Autodesk Inventor part; units mm, degrees
ref_plane "YZ Plane" through (0, 0, 0) normal (1, 0, 0) x (0, 1, 0)
ref_plane "XZ Plane" through (0, 0, 0) normal (0, 1, 0) x (-1, 0, 0)
ref_plane "XY Plane" through (0, 0, 0) normal (0, 0, 1) x (1, 0, 0)
sketch "Sketch1" plane through (0, 0, 0) normal (0, 0, 1) x (1, 0, 0)
  circle A0 centre (0, 12.7) radius 1.5875
  circle A1 centre (-0.0751, 0) radius 1.5875
  line L0 (-0.0751, 0) -> (-0.0751, 19.0499)
  line L1 (-0.0751, 1.5875) -> (-0.0751, 24.8386)
  line L2 (6.35, 15.5543) -> (6.35, 5.2605)
  line L3 (9.525, 2.0855) -> (15.8376, 2.0855)
  line L4 (-6.5001, 15.5229) -> (-6.5001, 5.2772)
  line L5 (-9.6751, 2.1022) -> (-15.8387, 2.1022)
  arc A2 (-19.0064, -1.2874) -> (19.0051, -1.3074) centre (0, 0) ccw
  arc A3 (3.81, 18.6651) -> (-3.9901, 18.6274) centre (0, 0) ccw
  arc A4 (-3.9901, 18.6274) -> (-6.5001, 15.5229) centre (-3.3251, 15.5229) ccw
  arc A5 (6.35, 15.5543) -> (3.81, 18.6651) centre (3.175, 15.5543) ccw
  arc A6 (6.35, 5.2605) -> (9.525, 2.0855) centre (9.525, 5.2605) ccw
  arc A7 (-9.6751, 2.1022) -> (-6.5001, 5.2772) centre (-9.6751, 5.2772) ccw
  arc A8 (-15.8387, 2.1022) -> (-19.0064, -1.2874) centre (-15.8387, -1.0728) ccw
  arc A9 (19.0051, -1.3074) -> (15.8376, 2.0855) centre (15.8376, -1.0895) ccw
  point P0 (6.35, 17.9605)
  point P1 (6.35, 2.0855)
  point P2 (18.9355, 2.0855)
  point P3 (-6.5001, 2.1022)
  point P4 (-18.9337, 2.1022)
  point P5 (-6.5001, 17.9067)
  dimension "d6" = 3.175
  dimension "d3" = 3.175
  dimension "d11" = 15.875
  dimension "d12" = 3.175
extrude "Extrusion1" add sketch "Sketch1" along normal blind 12.7
properties part number "Crank Cutting Jig"
Build history of the part. All positions in model axes, mm. A direction names the side the tool comes from. Coordinates: 2 decimals unless noted, no trailing zeros. Write each loop counter-clockwise with the first axis right and the second up, starting at its lowest first coordinate (ties: lowest second). Pieces come first, ordered by that corner, then holes.
(1) 3-axis set-ups, long thin cutter, end or side, ignore diameter. For faces 4 (the cylindrical face through (0.391, -19.046, 6.261)), 5 (the flat face through (-6.5, 10, 6)), 6 (the flat face through (13, 2.086, 6)): which of +Z, -Z, +X, -X, +Y, -Y reach the whole face in a straight line?
(2) Cut at B-B on z = 7. State how many separate pieces and enclosed holes the cut face has, and give its area (3 significant figures).
(3) Cut at C-C on x = 0. List the corners of the cut face in (y, z), and give its area (3 significant figures).
(4) Pin check, flat tips, straight feed: pin 1 Ø1.5 at (y, z) = (-5.5, 9.5) entering from -X; pin 2 Ø5 at (x, y) = (0, 12.7) entering from -Z; pin 3 Ø4 at (x, y) = (10, 8.5) entering from +Z; pin 4 Ø5 at (y, z) = (9.5, 4.5) entering from -X. Stop position of each tip, or through.
(5) Mould opens along X. For faces 1 (the cylindrical face through (7.305, 2.991, 6.261)), 2 (the flat face through (-13, 2.102, 6)), 3 (the cylindrical face through (1.44, -0.48, 6.26)) say: pulls with the +X half, pulls with the -X half, needs draft (parallel to the pull), parting line crosses it, or undercut.
(6) Cut at D-D on y = 0. List the corners of the cut face in (x, z).
(7) Cut at A-A on y = 12.7. List the corners of the cut face in (x, z), and give its area (3 significant figures).
(8) Drill centre lines: line 1 (Y direction, x = 0, z = 7.5); line 2 (X direction, y = 12.7, z = 2.75); line 3 (Y direction, x = 1, z = 8). Where is each one in solid material? Low to high.
Working result:
1. face 4: +Z, -Z, -Y
1. face 5: +Z, -Z, -X, +Y
1. face 6: +Z, -Z, +X, +Y
2. separate pieces: 1
2. enclosed holes: 2
2. area: 845 mm2
3. outline: (-19.05, 0) - (-1.59, 0) - (-1.59, 12.7) - (-19.05, 12.7) - close; (1.59, 0) - (11.11, 0) - (11.11, 12.7) - (1.59, 12.7) - close; (14.29, 0) - (19.05, 0) - (19.05, 12.7) - (14.29, 12.7) - close
3. area: 403 mm2
4. pin 1: stops at x = -18.45
4. pin 2: stops at z = 0
4. pin 3: passes through
4. pin 4: stops at x = -6.5
5. face 1: pulls with the +X half
5. face 2: needs draft
5. face 3: undercut
6. outline: (-18.83, 0) - (-1.66, 0) - (-1.66, 12.7) - (-18.83, 12.7) - close; (1.51, 0) - (18.82, 0) - (18.82, 12.7) - (1.51, 12.7) - close
7. outline: (-6.5, 0) - (-1.59, 0) - (-1.59, 12.7) - (-6.5, 12.7) - close; (1.59, 0) - (6.35, 0) - (6.35, 12.7) - (1.59, 12.7) - close
7. area: 123 mm2
8. line 1: y = -19.05 to -1.59, 1.59 to 11.11, 14.29 to 19.05
8. line 2: x = -6.5 to -1.59, 1.59 to 6.35
8. line 3: y = -19.02 to -1.17, 1.17 to 11.47, 13.93 to 19.02
